Verification items for the finished model (mm, model axes). Round coordinates to 2 decimals unless told otherwise and drop trailing zeros. Write each loop counter-clockwise with the first axis right and the second up, starting at its lowest first coordinate (ties: lowest second). Pieces come first, ordered by that corner, then holes. Notation, with made-up numbers: M 65,-40 L 91,-40 A38 cw 91,-1 Z; hole C 40,52 d10. An arc over 180 degrees is marked long. One line per question, with ' | ' between items. Start each with the question number.
Q1. Cross-section at A-A (z = 28). Record the boundary of the cut face in (x, y).
Q2. Cross-section at D-D (y = -213). Record the boundary of the cut face in (x, z), then the cut area to 3 significant figures.
Q3. Cross-section at C-C (y = -158). Record the boundary of the cut face in (x, z), then the cut area to 3 significant figures.
Q4. Cross-section at B-B (x = -52). Record the boundary of the cut face in (y, z).
Q5. Thickness scan on line 1 along Y through (x, z) = (-45.5, 27); line 2 along Z through (x, y) = (-69, -46.5); line 3 along Y through (x, z) = (-49, 36). Record the ranges inside material, lowest first. Write a range as from..to.
Q6. Gauge pin test, flat ends, axial feed: pin 1 (3 mm diameter, centred on x = -71, z = 18.5, fed in from +Y); pin 2 (5 mm diameter, centred on x = -52, z = 27, fed in from -Y); pin 3 (1 mm diameter, centred on x = -90, z = 16.5, fed in from +Y). Record the tip position at first contact, or that the pin passes through.
from build123d import *

# Parameters (mm, degrees)
F0_W     = 100.2259999514
F0_H     = 20.5646064132
F1_DEPTH = 230
F2_R     = 5
F3_W     = 20.0339406729
F3_H     = 179.7797265649
F4_DEPTH = 40
F5_R     = 30
F6_W     = 147.0367200673
F6_H     = 24.7304122895
F7_DEPTH = 25
F8_R     = 15
F9_R     = 5
F10_SIZE = 2
F11_SIZE = 2


with BuildPart() as f1:
    # F0 (on Front) → F1 (new body)
    with BuildSketch(Plane.XZ):
        with Locations((-50.1129999757, 10.2823032066)):
            Rectangle(F0_W, F0_H)
    extrude(amount=F1_DEPTH)

    # F2
    f2_edges = [f1.edges().sort_by_distance(p)[0] for p in [
        (-50.113, -230, 20.564606),
        (0, -115, 20.564606),
        (-100.226, -115, 20.564606),
        (-50.113, 0, 20.564606),
    ]]
    fillet(f2_edges, radius=F2_R)

    # F3 (on face) → F4 (join)
    with BuildSketch(Plane.XY.offset(20.5646064132)):
        with Locations((-50.1129999757, -115)):
            Rectangle(F3_W, F3_H)
    extrude(amount=F4_DEPTH)

    # F5
    f5_edges = [f1.edges().sort_by_distance(p)[0] for p in [
        (-50.113, -25.110137, 60.564606),
        (-50.113, -204.889863, 60.564606),
    ]]
    fillet(f5_edges, radius=F5_R)

    # F6 (on face) → F7 (cut)
    with BuildSketch(Plane(origin=(-60.1299703121, 0, 0), x_dir=(0, -1, 0), z_dir=(-1, 0, 0))):
        with Locations((114.8098763078, 32.929812558)):
            Rectangle(F6_W, F6_H)
    extrude(amount=-F7_DEPTH, mode=Mode.SUBTRACT)

    # F8
    f8_edges = [f1.edges().sort_by_distance(p)[0] for p in [
        (-50.113, -188.328236, 45.295019),
        (-50.113, -41.291516, 45.295019),
    ]]
    fillet(f8_edges, radius=F8_R)

    # F9
    f9_edges = [f1.edges().sort_by_distance(p)[0] for p in [
        (-60.12997, -115, 60.564606),
        (-60.12997, -33.896933, 51.77781),
        (-60.12997, -114.809876, 45.295019),
        (-60.12997, -45.684915, 40.90162),
        (-60.12997, -183.934838, 40.90162),
        (-40.09603, -115, 60.564606),
        (-40.09603, -196.103067, 51.77781),
        (-40.09603, -114.809876, 45.295019),
    ]]
    fillet(f9_edges, radius=F9_R)

    # F10
    f10_edges = [f1.edges().sort_by_distance(p)[0] for p in [
        (-50.113, -230, 0),
    ]]
    chamfer(f10_edges, length=F10_SIZE)

    # F11
    f11_edges = [f1.edges().sort_by_distance(p)[0] for p in [
        (-50.113, 0, 0),
    ]]
    chamfer(f11_edges, length=F11_SIZE)


solid = f1.part
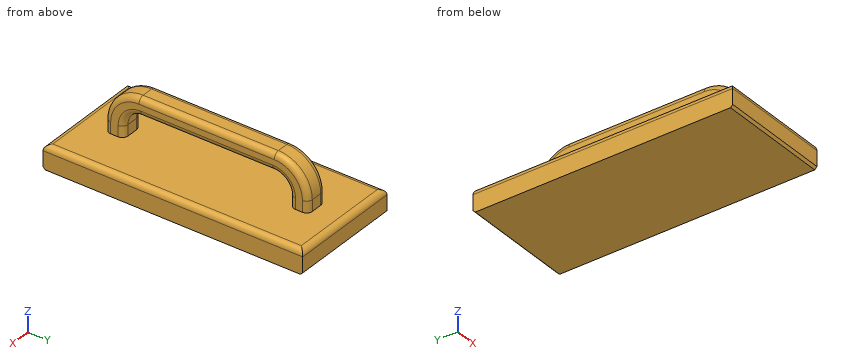
Determined:
1) outline: M -60.13,-199.89 A5 ccw -55.13,-204.89 L -45.1,-204.89 A5 ccw -40.1,-199.89 L -40.1,-193.33 A5 ccw -45.1,-188.33 L -55.13,-188.33 A5 ccw -60.13,-193.33 Z; M -60.13,-36.29 A5 ccw -55.13,-41.29 L -45.1,-41.29 A5 ccw -40.1,-36.29 L -40.1,-30.11 A5 ccw -45.1,-25.11 L -55.13,-25.11 A5 ccw -60.13,-30.11 Z
2) outline: M -100.23,0 L 0,0 L 0,15.56 A5 ccw -5,20.56 L -95.23,20.56 A5 ccw -100.23,15.56 Z | area: 2,050 mm²
3) outline: M -100.23,0 L 0,0 L 0,15.56 A5 ccw -5,20.56 L -95.23,20.56 A5 ccw -100.23,15.56 Z; M -60.13,50.3 A5 ccw -55.13,45.3 L -45.1,45.3 A5 ccw -40.1,50.3 L -40.1,55.56 A5 ccw -45.1,60.56 L -55.13,60.56 A5 ccw -60.13,55.56 Z | area: 2,330 mm²
4) outline: M -230,2 L -228,0 L -2,0 L 0,2 L 0,15.56 A5 ccw -5,20.56 L -25.11,20.56 L -25.11,30.56 A30 ccw -55.11,60.56 L -174.89,60.56 A30 ccw -204.89,30.56 L -204.89,20.56 L -225,20.56 A5 ccw -230,15.56 Z; hole M -188.33,20.56 L -41.29,20.56 L -41.29,30.3 A15 ccw -56.29,45.3 L -173.33,45.3 A15 ccw -188.33,30.3 Z
5) line 1: y = -204.89..-188.33, -41.29..-25.11 | line 2: z = 0..20.56 | line 3: y = -204.39..-187.2, -42.42..-25.61
6) pin 1: stops at y = -0.21 | pin 2: stops at y = -204.89 | pin 3: stops at y = -0.02
